```python
from build123d import *

# Parameters (mm, degrees)
SKETCH1_R           = 1
BOSS_EXTRUDE1_DEPTH = 9.2
SKETCH2_R           = 1.5
BOSS_EXTRUDE2_DEPTH = 0.5
SKETCH4_W           = 0.2
SKETCH4_H           = 0.32


with BuildPart() as part:
    # Sketch1 → Boss-Extrude1 (new body)
    with BuildSketch(Plane(origin=(0, 0, 0), x_dir=(1, 0, 0), z_dir=(0, 1, 0))):
        with Locations(Location((0, 0, 0), (0, 0, 270))):
            Circle(SKETCH1_R)
    extrude(amount=BOSS_EXTRUDE1_DEPTH)

    # Sketch2 → Boss-Extrude2 (add)
    with BuildSketch(Plane(origin=(0, 9.2, 0), x_dir=(1, 0, 0), z_dir=(0, 1, 0))):
        with Locations(Location((0, 0, 0), (0, 0, 270))):
            Circle(SKETCH2_R)
    extrude(amount=BOSS_EXTRUDE2_DEPTH)

    # Sketch4 → Cut-Revolve4 (revolve, cut)
    with BuildSketch(Plane(origin=(0, 0, 0), x_dir=(0, 0, -1), z_dir=(1, 0, 0))):
        with Locations((-0.9, 0.39)):
            Rectangle(SKETCH4_W, SKETCH4_H)
    revolve(axis=Axis((0, 9.2, 0), (0, -1, 0)), mode=Mode.SUBTRACT)


solid = part.part
```
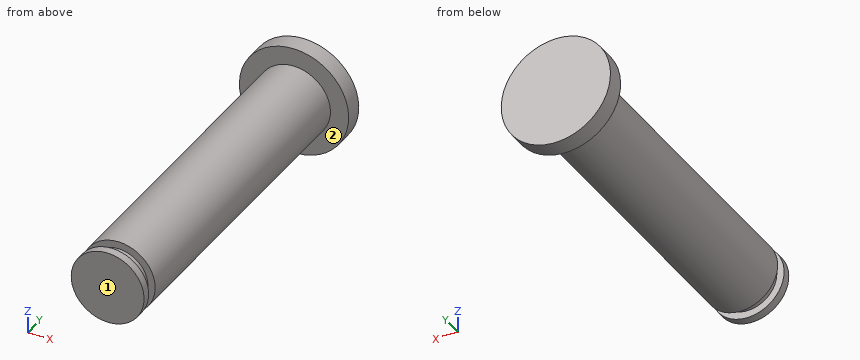
Could you check a few things on this model? Use its own coordinates, in mm. Face numbers are marked on the shaded views. A direction names the side the tool comes from. Coordinates: 2 decimals unless noted, no trailing zeros. Order: outer loops, then holes, each group sorted by start corner. A loop starts at its lowest first (then second) coordinate and runs counter-clockwise, first axis right, second up. Notation, with made-up numbers: M 52,62.5 L 104,62.5 A17 cw 104,95.5 Z; hole C 43.25,-15 d2. An arc over 180 degrees is marked long. Use one line per item in the form item = value. Start each with the question number.
1. Suppose I cut it at C-C on y = 2.5. Write out the boundary of the cut face in (x, z).
2. Please list where these lines run through material, in increasing order: line 1 (Y direction, x = 0.6, z = 1.05); line 2 (X direction, y = 6.75, z = -0.05); line 3 (X direction, y = 2.25, z = 0.35).
3. On a 3-axis mill with a long thin cutter (end or side, diameter ignored), from which of +Z, -Z, +X, -X, +Y, -Y can I reach the whole of each face in a straight line? I mean the marked faces 1 and 2. Say none if no direction works.
4. Suppose I cut it at A-A on z = -0.9. Write out the boundary of the cut face in (x, y).
5. Suppose I cut it at B-B on x = 0. Write out the boundary of the cut face in (y, z), then the cut area to 3 significant figures.
6. Suppose I cut it at D-D on z = 0. Write out the boundary of the cut face in (x, y), then the cut area to 3 significant figures.
Geometry says:
q1.outline = C 0,0 d2
q2.line_1 = 9.2 to 9.7
q2.line_2 = -1 to 1
q2.line_3 = -0.94 to 0.94
q3.face_1 = +Z, -Z, +X, -X, -Y
q3.face_2 = -Y
q4.outline = M -1.2,9.2 L -0.44,9.2 L -0.44,0.55 L 0.44,0.55 L 0.44,9.2 L 1.2,9.2 L 1.2,9.7 L -1.2,9.7 Z; M -0.44,0 L 0.44,0 L 0.44,0.23 L -0.44,0.23 Z
q5.outline = M 0,-1 L 0.23,-1 L 0.23,-0.8 L 0.55,-0.8 L 0.55,-1 L 9.2,-1 L 9.2,-1.5 L 9.7,-1.5 L 9.7,1.5 L 9.2,1.5 L 9.2,1 L 0.55,1 L 0.55,0.8 L 0.23,0.8 L 0.23,1 L 0,1 Z
q5.area = 19.8 mm^2
q6.outline = M -1.5,9.2 L -1,9.2 L -1,0.55 L -0.8,0.55 L -0.8,0.23 L -1,0.23 L -1,0 L 1,0 L 1,0.23 L 0.8,0.23 L 0.8,0.55 L 1,0.55 L 1,9.2 L 1.5,9.2 L 1.5,9.7 L -1.5,9.7 Z
q6.area = 19.8 mm^2
